from build123d import *

# Parameters (mm, degrees)
BOSS_EXTRUDE1_DEPTH = 137.5
SKETCH3_W           = 20
SKETCH3_H           = 12.2
BOSS_EXTRUDE2_DEPTH = 2
SKETCH2_W           = 4.4
SKETCH2_H           = 261
CUT_EXTRUDE1_DEPTH  = 13.2
FILLET3_R           = 2
CHAMFER1_SIZE       = 1
SKETCH4_W           = 10.203047284
SKETCH4_H           = 4
CUT_EXTRUDE2_DEPTH  = 2.5
LPATTERN2_COUNT     = 2
LPATTERN2_PITCH     = 33
BOSS_EXTRUDE3_START = -275
SKETCH7_W           = 13
SKETCH7_H           = 12.2
BOSS_EXTRUDE3_DEPTH = 275
SKETCH8_W           = 275
SKETCH8_H           = 12.2
BOSS_EXTRUDE4_DEPTH = 15
M4_TAPPED_HOLE1_D   = 3.3
LPATTERN3_COUNT     = 4
LPATTERN3_PITCH     = 78.333333333
MIRROR5_COPY_1_D    = 3.3
MIRROR5_COPY_2_D    = 3.3
MIRROR5_COPY_3_D    = 3.3
M4_TAPPED_HOLE2_D   = 3.3
FILLET1_R           = 1.5
CHAMFER2_SIZE       = 0.5
CHAMFER4_SIZE       = 2
FILLET4_R           = 1
M4_TAPPED_HOLE3_D   = 3.3


with BuildPart() as part:
    # Sketch1 → Boss-Extrude1 (new body, symmetric)
    with BuildSketch(Plane.XY):
        Polygon((-10, -2.7), (-10, 9.5), (10, 9.5), (10, -2.7), (8, -2.7), (8, 2.5), (4.2, 2.5), (4.2, 0), (-4.2, 0), (-4.2, 2.5), (-8, 2.5), (-8, -2.7), align=None)
    extrude(amount=BOSS_EXTRUDE1_DEPTH, both=True)

    # Sketch3 → Boss-Extrude2 (add)
    with BuildSketch(Plane.XY.offset(137.5)):
        with Locations((0, 3.4)):
            Rectangle(SKETCH3_W, SKETCH3_H)
    boss_extrude2 = extrude(amount=-BOSS_EXTRUDE2_DEPTH)

    # Mirror1: Boss-Extrude2 across plane
    add(boss_extrude2.mirror(Plane.XY))

    # Sketch2 → Cut-Extrude1 (cut, through all)
    with BuildSketch(Plane(origin=(0, 9.5, 0), x_dir=(1, 0, 0), z_dir=(0, 1, 0))):
        Rectangle(SKETCH2_W, SKETCH2_H)
    extrude(amount=-CUT_EXTRUDE1_DEPTH, mode=Mode.SUBTRACT)

    # Fillet3
    fillet3_edges = [part.edges().sort_by_distance(p)[0] for p in [
        (2.2, 4.75, -130.5),
        (2.2, 4.75, 130.5),
        (-2.2, 4.75, 130.5),
        (-2.2, 4.75, -130.5),
    ]]
    fillet(fillet3_edges, radius=FILLET3_R)

    # Chamfer1
    chamfer1_edges = [part.edges().sort_by_distance(p)[0] for p in [
        (-2.2, 0, 0),
        (0, 0, -130.5),
        (2.2, 0, 0),
        (0, 0, 130.5),
        (-1.614213562, 0, -129.914213562),
        (1.614213562, 0, -129.914213562),
        (1.614213562, 0, 129.914213562),
        (-1.614213562, 0, 129.914213562),
    ]]
    chamfer(chamfer1_edges, length=CHAMFER1_SIZE)

    # Sketch4 → Cut-Extrude2 (cut)
    with BuildSketch(Plane.XZ):
        with Locations((-0.901523642, 133.5)):
            Rectangle(SKETCH4_W, SKETCH4_H)
    cut_extrude2 = extrude(amount=-CUT_EXTRUDE2_DEPTH, mode=Mode.SUBTRACT)

    # Mirror2: Cut-Extrude2 across plane
    add(cut_extrude2.mirror(Plane.XY), mode=Mode.SUBTRACT)


with BuildPart() as lpattern2_1:
    # LPattern2: pattern copy
    add(part.part.moved(Location(Vector(1, 0, 0) * (1 * LPATTERN2_PITCH))))


with BuildPart() as part_1:
    add(part.part)

    add(lpattern2_1.part)  # Boss-Extrude3 merges LPattern2_1
    # Sketch7 → Boss-Extrude3 (add)
    with BuildSketch(Plane(origin=(0, 0, -137.5), x_dir=(-1, 0, 0), z_dir=(0, 0, -1)).offset(BOSS_EXTRUDE3_START)):
        with Locations((-16.5, 3.4)):
            Rectangle(SKETCH7_W, SKETCH7_H)
    extrude(amount=BOSS_EXTRUDE3_DEPTH)

    # Sketch8 → Boss-Extrude4 (add)
    with BuildSketch(Plane.ZY.offset(10)):
        with Locations((0, 3.4)):
            Rectangle(SKETCH8_W, SKETCH8_H)
    boss_extrude4 = extrude(amount=BOSS_EXTRUDE4_DEPTH)

    # Mirror4: Boss-Extrude4 across plane
    add(boss_extrude4.mirror(Plane.ZY.offset(-16.5)))

    # M4 Tapped Hole1 (through all)
    with Locations(Plane(origin=(0, 9.5, 0), x_dir=(1, 0, 0), z_dir=(0, 1, 0))):
        with Locations((-17, 117.5)):
            m4_tapped_hole1 = Hole(M4_TAPPED_HOLE1_D / 2)

    # LPattern3: M4 Tapped Hole1 ×4
    with Locations(*[(0, 0, i * LPATTERN3_PITCH) for i in range(1, LPATTERN3_COUNT)]):
        add(m4_tapped_hole1, mode=Mode.SUBTRACT)

    # Mirror5: M4 Tapped Hole1 across plane
    add(m4_tapped_hole1.mirror(Plane.ZY.offset(-16.5)), mode=Mode.SUBTRACT)

    # Mirror5 copy 1 (through all)
    with Locations(Plane(origin=(33, 9.5, 78.333333333), x_dir=(-1, 0, 0), z_dir=(0, 1, 0))):
        with Locations((-17, -117.5)):
            Hole(MIRROR5_COPY_1_D / 2)

    # Mirror5 copy 2 (through all)
    with Locations(Plane(origin=(33, 9.5, 156.666666667), x_dir=(-1, 0, 0), z_dir=(0, 1, 0))):
        with Locations((-17, -117.5)):
            Hole(MIRROR5_COPY_2_D / 2)

    # Mirror5 copy 3 (through all)
    with Locations(Plane(origin=(33, 9.5, 235), x_dir=(-1, 0, 0), z_dir=(0, 1, 0))):
        with Locations((-17, -117.5)):
            Hole(MIRROR5_COPY_3_D / 2)

    # M4 Tapped Hole2 (through all)
    with Locations(Plane(origin=(0, 9.5, 0), x_dir=(1, 0, 0), z_dir=(0, 1, 0))):
        with Locations((52.741079456, -70.992499999), (52.741079456, 71.007500001)):
            Hole(M4_TAPPED_HOLE2_D / 2)

    # Fillet1
    fillet1_edges = [part_1.edges().sort_by_distance(p)[0] for p in [
        (41, -0.1, 135.5),
        (25, -0.1, 135.5),
        (41, -0.1, -135.5),
        (25, -0.1, -135.5),
        (-8, -0.1, 135.5),
        (8, -0.1, 135.5),
        (-8, -0.1, -135.5),
        (8, -0.1, -135.5),
    ]]
    fillet(fillet1_edges, radius=FILLET1_R)

    # Chamfer2
    chamfer2_edges = [part_1.edges().sort_by_distance(p)[0] for p in [
        (33, -2.7, -135.5),
        (41, -2.7, 0),
        (25, -2.7, 0),
        (33, -2.7, 135.5),
        (0, -2.7, -135.5),
        (-8, -2.7, 0),
        (8, -2.7, 0),
        (0, -2.7, 135.5),
        (40.560660172, -2.7, -135.060660172),
        (25.439339828, -2.7, -135.060660172),
        (40.560660172, -2.7, 135.060660172),
        (25.439339828, -2.7, 135.060660172),
        (-7.560660172, -2.7, -135.060660172),
        (7.560660172, -2.7, -135.060660172),
        (7.560660172, -2.7, 135.060660172),
        (-7.560660172, -2.7, 135.060660172),
    ]]
    chamfer(chamfer2_edges, length=CHAMFER2_SIZE)

    # Chamfer4
    chamfer4_edges = [part_1.edges().sort_by_distance(p)[0] for p in [
        (-25, 3.4, -137.5),
        (-25, 3.4, 137.5),
        (58, 3.4, 137.5),
        (58, 3.4, -137.5),
    ]]
    chamfer(chamfer4_edges, length=CHAMFER4_SIZE)

    # Fillet4
    fillet4_edges = [part_1.edges().sort_by_distance(p)[0] for p in [
        (-4.2, 1.25, 131.5),
        (4.2, 1.25, 131.5),
        (-4.2, 1.25, -131.5),
        (4.2, 1.25, -131.5),
        (28.8, 1.25, 131.5),
        (37.2, 1.25, 131.5),
        (28.8, 1.25, -131.5),
        (37.2, 1.25, -131.5),
    ]]
    fillet(fillet4_edges, radius=FILLET4_R)

    # M4 Tapped Hole3 (through all)
    with Locations(Plane(origin=(0, 9.5, 0), x_dir=(1, 0, 0), z_dir=(0, 1, 0))):
        with Locations((-18.158920544, -70.992499999), (-18.158920544, 71.007500001)):
            Hole(M4_TAPPED_HOLE3_D / 2)


solid = part_1.part
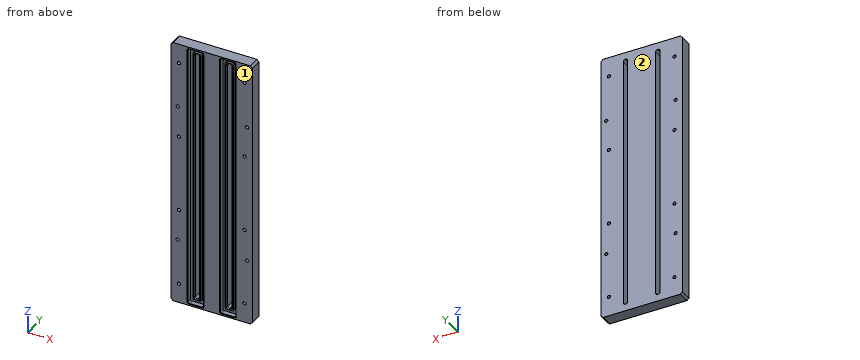
Can you work these out from the model? Positions are in its coordinate system, mm. Face numbers are marked on the shaded views. Coordinates: 2 decimals unless noted, no trailing zeros. Write item = value, one per line.
(1) If we mould it in two halves opening along Y, with no side actions, what happens to the marked faces 1 and 2? For each: pulls with the +Y half, pulls with the -Y half, needs draft (parallel to the pull), parting line crosses it, or undercut.
Results are:
face_1 = pulls with the -Y half
face_2 = pulls with the +Y half
(2) I need wall thicknesses on line 1 along X through (y, z) = (3.5, -77.5); line 2 along X through (y, z) = (-2, -29); line 3 along Z through (x, y) = (50, 1.5). Which ranges of each line are inside material? Lowest first, please. Write a range as [from, to].
Results are:
line_1 = [-25, -2.2], [2.2, 30.8], [35.2, 58]
line_2 = [-25, -8], [8, 25], [41, 58]
line_3 = [-137.5, -119.15], [-115.85, -40.82], [-37.52, 37.52], [40.82, 115.85], [119.15, 137.5]
(3) Suppose I cut it at A-A on z = -83.5. State how many separate pieces and enclosed holes the cut face has, plus the area to 3 significant figures.
Results are:
separate_pieces = 3
enclosed_holes = 0
area = 802 mm2
(4) For pin 1 Ø2.5 at (x, z) = (50, -39.17) entering from +Y; pin 2 Ø2 at (x, z) = (31.5, -11) entering from -Y, each with a flat end and sliding along its axis, tell me the tip position at first contact or that it passes through.
Results are:
pin_1 = through
pin_2 = 0.7
